Read the model definition and answer for the solid it produces. Units are mm, in the model's axes. A direction names the side the tool comes from. Give positions to 0.01 mm unless a question says otherwise; leave off trailing zeros. Order: outer loops, then holes, each group sorted by start corner. A loop starts at its lowest first (then second) coordinate and runs counter-clockwise, first axis right, second up. Notation, with made-up numbers: (79, -14.5) -> (101, -14.5) arc R16 cw to (101, -8.5) -> close; hole circle Ø7 at (-22, 42.25). An arc over 180 degrees is marked (long way). Use one line per item in the form item = value.
```python
from build123d import *

# Parameters (mm, degrees)
SKETCH_R     = 42
PAD_DEPTH    = 7
SKETCH003_R  = 27
PAD001_DEPTH = 25
SKETCH004_R  = 3
HOLE_DEPTH   = 25


with BuildPart() as part:
    # Sketch → Pad (new body)
    with BuildSketch(Plane.XY):
        Circle(SKETCH_R)
        with BuildLine():
            Line((-2.9, 14.895322), (-2.9, 12.895322))
            Line((-2.9, 12.895322), (2.9, 12.895322))
            Line((2.9, 12.895322), (2.9, 14.895322))
            ThreePointArc((-2.9, 14.895322), (0, -15.175), (2.9, 14.895322))
        make_face(mode=Mode.SUBTRACT)
    extrude(amount=PAD_DEPTH)

    # Sketch003 (on Face7 of Pad) → Pad001 (join)
    with BuildSketch(Plane.XY.offset(7)):
        Circle(SKETCH003_R)
        with BuildLine():
            ThreePointArc((-2.9, 14.895322), (0, -15.175), (2.9, 14.895322))
            Line((2.9, 12.895322), (2.9, 14.895322))
            Line((-2.9, 12.895322), (2.9, 12.895322))
            Line((-2.9, 14.895322), (-2.9, 12.895322))
        make_face(mode=Mode.SUBTRACT)
    extrude(amount=PAD001_DEPTH)

    # Sketch004 (on Face3 of Pad001) → Hole (cut)
    with BuildSketch(Plane.XY.offset(7)):
        with Locations((0, 32.5)):
            Circle(SKETCH004_R)
        with Locations((0, -32.5)):
            Circle(SKETCH004_R)
        with Locations((32.5, 0)):
            Circle(SKETCH004_R)
        with Locations((-32.5, 0)):
            Circle(SKETCH004_R)
    extrude(amount=-HOLE_DEPTH, mode=Mode.SUBTRACT)


solid = part.part
```
Item 1: Determine the mould class of faces 4 (the cylindrical face through (29.5, 0.1, 3.5)), 5 (the cylindrical face through (-0.65, -35.43, 3.55)), 6 (the flat face through (18, 1, 0)), 7 (the cylindrical face through (40.06, 12.62, 3.45)) for opening direction X: +X half, -X half, draft (parallel to the pull), parting line (faces both ways), or undercut.
Checks:
face_4 = undercut
face_5 = undercut
face_6 = draft
face_7 = parting line
Item 2: Straight lines are drawn through the part: L1, parallel to Y at x = 0, z = 4 (3 decimals); L2, parallel to Z at x = 30, y = 8.5; L3, parallel to Y at x = 5, z = 29. For each, find the intervals that lie inside material, in ascending order. Write a range as from..to.
Checks:
L1 = -42..-35.5, -29.5..-15.175, 12.895..29.5, 35.5..42
L2 = 0..7
L3 = -26.53..-14.33, 14.33..26.53
Item 3: The part is cut by section A-A on y = 0. Give the vertices of the cut face in (x, z) (3 decimals).
Checks:
outline = (-42, 0) -> (-35.5, 0) -> (-35.5, 7) -> (-42, 7) -> close; (-29.5, 0) -> (-15.175, 0) -> (-15.175, 32) -> (-27, 32) -> (-27, 7) -> (-29.5, 7) -> close; (15.175, 0) -> (29.5, 0) -> (29.5, 7) -> (27, 7) -> (27, 32) -> (15.175, 32) -> close; (35.5, 0) -> (42, 0) -> (42, 7) -> (35.5, 7) -> close
Item 4: The part is cut by section B-B on x = 0. Give the vertices of the cut face in (y, z) (3 decimals), and give its area (3 significant figures).
Checks:
outline = (-42, 0) -> (-35.5, 0) -> (-35.5, 7) -> (-42, 7) -> close; (-29.5, 0) -> (-15.175, 0) -> (-15.175, 32) -> (-27, 32) -> (-27, 7) -> (-29.5, 7) -> close; (12.895, 0) -> (29.5, 0) -> (29.5, 7) -> (27, 7) -> (27, 32) -> (12.895, 32) -> close; (35.5, 0) -> (42, 0) -> (42, 7) -> (35.5, 7) -> close
area = 956 mm²
Item 5: Given pin 1 Ø0.6 at (y, z) = (14, 14) entering from -X; pin 2 Ø2 at (y, z) = (14.5, 15.5) entering from +X; pin 3 Ø4 at (x, y) = (32, 11.5) entering from +Z; pin 4 Ø12 at (x, y) = (-18, 22.5) entering from +Z, each flat-ended and moving along its own axis, determine where each tip first touches the part or whether it passes through.
Checks:
pin_1 = -23.27
pin_2 = 23.38
pin_3 = 7
pin_4 = 32
Item 6: Which of the six approach directions +Z, -Z, +X, -X, +Y, -Y give full straight-line access (tool end or side, diameter ignored) to faces 1 (the flat face through (-0.6, -27.4, 7)), 2 (the flat face through (12, -12, 32)), 3 (the flat face through (0, 12.895, 16))?
Checks:
face_1 = +Z
face_2 = +Z, +X, -X, +Y, -Y
face_3 = +Z, -Z
Item 7: The part is cut by section D-D on x = -32.5. Give the vertices of the cut face in (y, z), and give its area (3 significant figures).
Checks:
outline = (-26.6, 0) -> (-3, 0) -> (-3, 7) -> (-26.6, 7) -> close; (3, 0) -> (26.6, 0) -> (26.6, 7) -> (3, 7) -> close
area = 330 mm²
Item 8: The part is cut by section C-C on z = 5.5. Give the vertices of the cut face in (x, y) (3 decimals).
Checks:
outline = circle Ø84 at (0, 0); hole circle Ø6 at (-32.5, 0); hole circle Ø6 at (0, -32.5); hole circle Ø6 at (0, 32.5); hole (-2.9, 12.895) -> (-2.9, 14.895) arc R15.175 ccw (long way) to (2.9, 14.895) -> (2.9, 12.895) -> close; hole circle Ø6 at (32.5, 0)
